Job drawing, mm, ordinate dimensions from the low corner. One solid piece. A direction names the side the tool comes from. Give positions to 0.01 mm unless a question says otherwise; leave off trailing zeros. Write each loop counter-clockwise with the first axis right and the second up, starting at its lowest first coordinate (ties: lowest second). Pieces come first, ordered by that corner, then holes. Notation, with made-up numbers: (84, 49.25) -> (101, 49.25) arc R19 cw to (101, 57.25) -> close; hole circle Ø4 at (27, 44). An arc over 180 degrees is marked (long way). Put each result on its own line as item: value. Start each with the question number.
Item 1: Tool access for the marked faces 1 and 2: list every direction of +Z, -Z, +X, -X, +Y, -Y with a clear straight run to the whole face (end or side of a thin tool).
Item 2: Slice it at C-C, the plane x = 959.5. List the corners of the cut face in (y, z), plus the area to 3 significant figures.
Item 3: Flat gauge pin, fed straight in: pin 1 Ø3 at (x, y) = (1262, 437.5) entering from -Z. Where does the tip first touch, or does it go through?
Item 4: Drill centre lines: line 1 along Z through (x, y) = (671, 101.5); line 2 along X through (y, z) = (393.5, 152). Where is each one in solid material? Low to high.
Item 5: Slice it at B-B, the plane z = 420. List the corners of the cut face in (x, y), plus the area to 3 significant figures.
Item 6: Slice it at A-A, the plane y = 102. List the corners of the cut face in (x, z), plus the area to 3 significant figures.
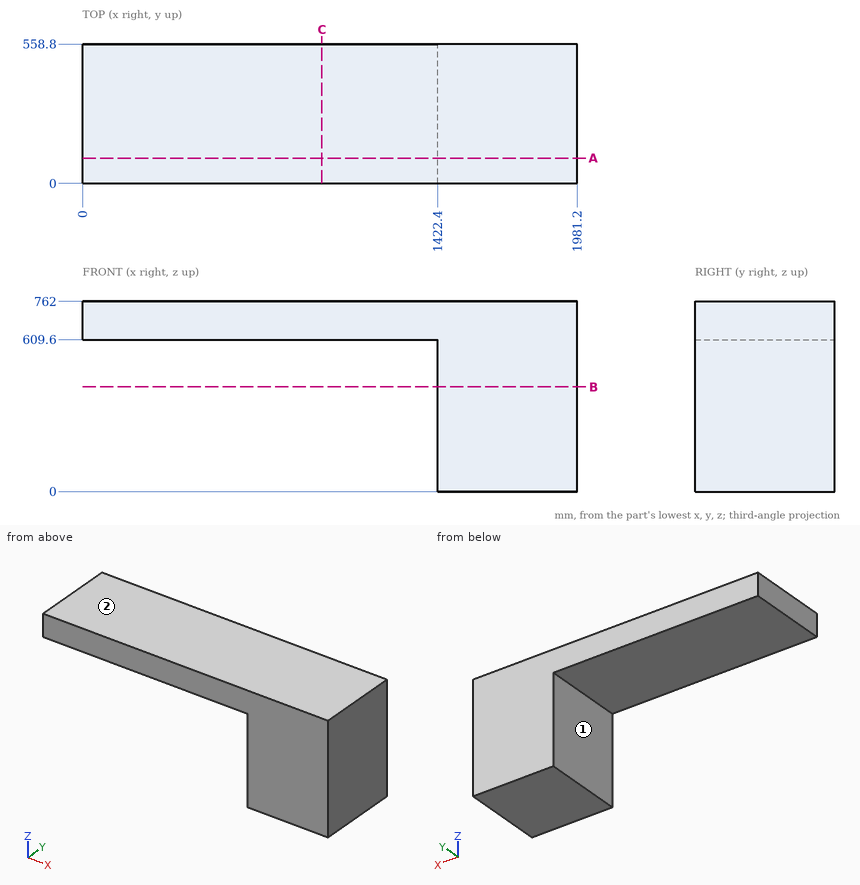
Values follow:
1. face 1: -Z, -X, +Y, -Y
1. face 2: +Z, +X, -X, +Y, -Y
2. outline: (0, 609.6) -> (558.8, 609.6) -> (558.8, 762) -> (0, 762) -> close
2. area: 85,200 mm2
3. pin 1: z = 609.6
4. line 1: 609.6 to 762
4. line 2: 1422.4 to 1981.2
5. outline: (1422.4, 0) -> (1981.2, 0) -> (1981.2, 558.8) -> (1422.4, 558.8) -> close
5. area: 312,000 mm2
6. outline: (0, 609.6) -> (1422.4, 609.6) -> (1422.4, 0) -> (1981.2, 0) -> (1981.2, 762) -> (0, 762) -> close
6. area: 643,000 mm2
